```python
from build123d import *

# Parameters (mm, degrees)
SKETCH2_W           = 30.48
SKETCH2_H           = 30.48
BOSS_EXTRUDE1_DEPTH = 5.08
SKETCH3_R           = 5.588
BOSS_EXTRUDE2_DEPTH = 25.4
FILLET1_R           = 5.08


with BuildPart() as part:
    # Sketch2 → Boss-Extrude1 (new body)
    with BuildSketch(Plane(origin=(0, 0, 0), x_dir=(1, 0, 0), z_dir=(0, 1, 0))):
        with Locations((15.24, 15.24)):
            Rectangle(SKETCH2_W, SKETCH2_H)
    extrude(amount=BOSS_EXTRUDE1_DEPTH)

    # Sketch3 → Boss-Extrude2 (add)
    with BuildSketch(Plane(origin=(0, 5.08, 0), x_dir=(1, 0, 0), z_dir=(0, 1, 0))):
        with Locations(Location((15.24, 15.24, 0), (0, 0, 270))):
            Circle(SKETCH3_R)
    extrude(amount=BOSS_EXTRUDE2_DEPTH)

    # Sketch6 → Revolve1 (revolve)
    with BuildSketch(Plane(origin=(0, 30.48, 0), x_dir=(1, 0, 0), z_dir=(0, 1, 0))):
        with BuildLine():
            Line((15.24, 27.94), (15.24, 2.54))
            ThreePointArc((15.24, 2.54), (27.94, 15.24), (15.24, 27.94))
        make_face()
    revolve(axis=Axis((15.24, 30.48, -27.94), (0, 0, 1)))

    # Fillet1
    fillet1_edges = [part.edges().sort_by_distance(p)[0] for p in [
        (15.24, 5.08, -20.828),
        (15.24, 19.075428285, -20.828),
    ]]
    fillet(fillet1_edges, radius=FILLET1_R)


solid = part.part
```
Check sheet for the modelled part. Datum: model origin and axes. Units: mm. A direction names the side the tool comes from. Coordinates: 2 decimals unless noted, no trailing zeros. Loops run counter-clockwise (first coordinate to the right, second up) from the corner with the lowest first, then second, coordinate; pieces in that order, holes last.
1) Access from +Z, -Z, +X, -X, +Y, -Y to the whole of each face (thin tool, end or side, straight path). Record for faces 4 (the face through (12, 5.08, -26)), 5 (the face through (15, 3, 0)).
2) Gauge pin test, flat ends, axial feed: pin 1 (6 mm diameter, centred on x = 8, y = 36, fed in from +Z); pin 2 (10 mm diameter, centred on x = 15, y = 14.5, fed in from -Z); pin 3 (8 mm diameter, centred on x = 14, y = 35, fed in from -Z). Record the tip position at first contact, or that the pin passes through.
3) Release check for a two-part mould opening along Y. For faces 1 (the face through (30.48, 3, -15)), 2 (the face through (15, 0, -15)), 3 (the face through (9.785, 13.165, -16.451)) record: released by +Y, released by -Y, zero draft, split by the parting line, or undercut.
4) Sectioned sample at B-B (y = 26). Record the boundary of the cut face in (x, z), and give its area (3 significant figures).
5) Sectioned sample at A-A (x = 27). Record the boundary of the cut face in (y, z).
6) Material ranges on probe 1 along Y at (x, z) = (26.5, -18.5); probe 2 along Y at (x, z) = (26.5, -15.5); probe 3 along Y at (x, z) = (2.5, -28.5), recorded low to high.
Check sheet entries:
1. face 4: none
1. face 5: +Z, +X, -X, +Y, -Y
2. pin 1: stops at z = -4.1
2. pin 2: stops at z = -22
2. pin 3: stops at z = -27.92
3. face 1: zero draft
3. face 2: released by -Y
3. face 3: undercut
4. outline: circle Ø23.77 at (15.24, -15.24)
4. area: 444 mm2
5. outline: (0, -30.48) - (5.08, -30.48) - (5.08, 0) - (0, 0) - close; circle Ø9.59 at (30.48, -15.24)
6. probe 1: y = 0 to 5.08, 25.59 to 35.37
6. probe 2: y = 0 to 5.08, 24.61 to 36.35
6. probe 3: y = 0 to 5.08
